Geometry: final body of the model. Coordinates: model frame, mm. Face numbers are marked on the shaded views. A direction names the side the tool comes from. Give positions to 0.01 mm unless a question says otherwise; leave off trailing zeros. Loops run counter-clockwise (first coordinate to the right, second up) from the corner with the lowest first, then second, coordinate; pieces in that order, holes last. Notation, with made-up numbers: (89, -21) -> (99, -21) arc R26 ccw to (99, -6) -> close; hole circle Ø3 at (27, -13). An arc over 180 degrees is marked (long way). Answer in a Markdown table with one row per item. Add a question column.
1) Section query D-D (z = 3.25). Return the cut outline in (x, y), plus the area to 3 significant figures.
2) First-contact query: P1, Ø2, axis at x = -3, z = -7, coming from the +Y side; P2, Ø2, axis at x = 7.35, z = -3.16, coming from the +Y side; P3, Ø5, axis at x = 8.5, y = 14, coming from the -Z side. Flat tips, straight axial feed; report the tip coordinate or a pass-through.
3) Line query: line 1 (Y direction, x = 4.75, z = 1); line 2 (Y direction, x = 6.75, z = -2.25); line 3 (X direction, y = 38.5, z = 8.25). Output: solid intervals per line, ascending. Write a range as from..to.
4) Section query C-C (y = 27.5). Return the cut outline in (x, z).
5) Access query for the marked faces 1 and 2. Directions: +Z, -Z, +X, -X, +Y, -Y. A direction counts if a zero-diameter tool reaches every point of the face in a straight line with its end or side. Return the directions, or none.
```python
from build123d import *

# Parameters (mm, degrees)
SKETCH1_R           = 11.049
BOSS_EXTRUDE1_DEPTH = 40.9956
SKETCH2_R           = 5.0165
BOSS_EXTRUDE2_DEPTH = 2.032
SKETCH3_R           = 1.585
BOSS_EXTRUDE3_DEPTH = 9.271
SKETCH5_R           = 1.25
CUT_EXTRUDE4_DEPTH  = 3.175
SKETCH7_R           = 2.601
SKETCH7_R_2         = 2.093
CUT_EXTRUDE5_DEPTH  = 0.254


with BuildPart() as part:
    # Sketch1 → Boss-Extrude1 (new body)
    with BuildSketch(Plane(origin=(0, 0, 0), x_dir=(1, 0, 0), z_dir=(0, 1, 0))):
        with Locations(Location((0, 0, 0), (0, 0, 270))):
            Circle(SKETCH1_R)
    extrude(amount=BOSS_EXTRUDE1_DEPTH)

    # Sketch2 → Boss-Extrude2 (add)
    with BuildSketch(Plane(origin=(0, 40.9956, 0), x_dir=(1, 0, 0), z_dir=(0, 1, 0))):
        with Locations(Location((0, 0, 0), (0, 0, 270))):
            Circle(SKETCH2_R)
    extrude(amount=BOSS_EXTRUDE2_DEPTH)

    # Sketch3 → Boss-Extrude3 (add)
    with BuildSketch(Plane(origin=(0, 43.0276, 0), x_dir=(1, 0, 0), z_dir=(0, 1, 0))):
        with Locations(Location((0, 0, 0), (0, 0, 270))):
            Circle(SKETCH3_R)
    extrude(amount=BOSS_EXTRUDE3_DEPTH)

    # Sketch5 → Cut-Extrude4 (cut)
    with BuildSketch(Plane(origin=(0, 40.9956, 0), x_dir=(1, 0, 0), z_dir=(0, 1, 0))):
        with Locations(Location((-7.432335625, 2.959795122, 0), (0, 0, 270))):
            Circle(SKETCH5_R)
        with Locations(Location((-3.162563719, 7.348346122, 0), (0, 0, 270))):
            Circle(SKETCH5_R)
        with Locations(Location((2.959795122, 7.432335625, 0), (0, 0, 270))):
            Circle(SKETCH5_R)
        with Locations(Location((7.348346122, 3.162563719, 0), (0, 0, 270))):
            Circle(SKETCH5_R)
        with Locations(Location((7.432335625, -2.959795122, 0), (0, 0, 270))):
            Circle(SKETCH5_R)
        with Locations(Location((3.162563719, -7.348346122, 0), (0, 0, 270))):
            Circle(SKETCH5_R)
        with Locations(Location((-2.959795122, -7.432335625, 0), (0, 0, 270))):
            Circle(SKETCH5_R)
        with Locations(Location((-7.348346122, -3.162563719, 0), (0, 0, 270))):
            Circle(SKETCH5_R)
    extrude(amount=-CUT_EXTRUDE4_DEPTH, mode=Mode.SUBTRACT)

    # Sketch7 → Cut-Extrude5 (cut)
    with BuildSketch(Plane(origin=(0, 43.0276, 0), x_dir=(1, 0, 0), z_dir=(0, 1, 0))):
        with Locations(Location((0, 0, 0), (0, 0, 270))):
            Circle(SKETCH7_R)
        with Locations(Location((0, 0, 0), (0, 0, 270))):
            Circle(SKETCH7_R_2, mode=Mode.SUBTRACT)
    extrude(amount=-CUT_EXTRUDE5_DEPTH, mode=Mode.SUBTRACT)


solid = part.part
```
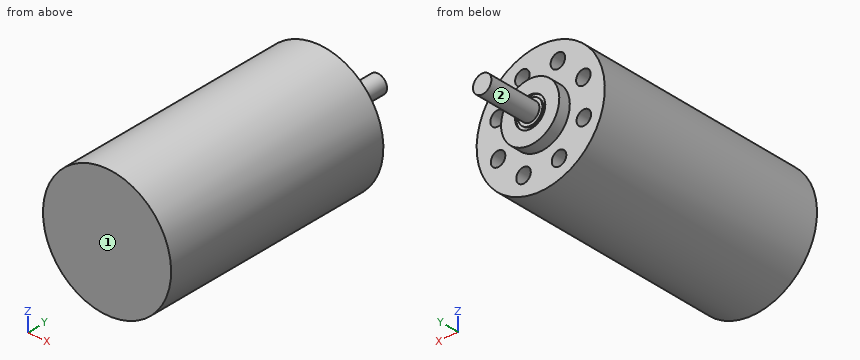
Evaluation:
| question | item | result |
|---|---|---|
| 1 | outline | (-10.56, 0) -> (10.56, 0) -> (10.56, 41) -> (8.65, 41) -> (8.65, 37.82) -> (6.22, 37.82) -> (6.22, 41) -> (3.82, 41) -> (3.82, 43.03) -> (-3.82, 43.03) -> (-3.82, 41) -> (-6.1, 41) -> (-6.1, 37.82) -> (-8.6, 37.82) -> (-8.6, 41) -> (-10.56, 41) -> close |
| 1 | area | 866 mm² |
| 2 | P1 | y = 41 |
| 2 | P2 | y = 37.82 |
| 2 | P3 | z = -9.28 |
| 3 | line 1 | 0..43.03 |
| 3 | line 2 | 0..37.82 |
| 3 | line 3 | -7.35..-3.91, -2.01..2.3, 4.03..7.35 |
| 4 | outline | circle Ø22.1 at (0, 0) |
| 5 | face 1 | +Z, -Z, +X, -X, -Y |
| 5 | face 2 | +Y |
